```python
from build123d import *

# Parameters (mm, degrees)
CHAMFER1_SIZE  = 0.5
CHAMFER1_SIZE2 = 0.3
CHAMFER2_SIZE  = 0.5
CHAMFER2_SIZE2 = 0.75


with BuildPart() as part:
    # Sketch1 → Revolve1 (revolve)
    with BuildSketch(Plane.XY):
        Polygon((3.75, 0), (3.75, 1.16), (1.6, 1.16), (1.6, 3.45), (0.625, 3.45), (0.625, 6.44), (2.645, 6.44), (2.645, 14.44), (3.095, 14.44), (3.095, 5.95), (1.6, 5.95), (1.6, 4.45), (3.09, 4.45), (3.09, 1.77), (4.5, 1.77), (4.5, 0), align=None)
    revolve(axis=Axis((0, 0, 0), (0, 1, 0)))

    # Chamfer1
    chamfer1_edges = [part.edges().sort_by_distance(p)[0] for p in [
        (-2.645, 14.44, 0),
    ]]
    chamfer1_side = [part.faces().sort_by_distance(p)[0] for p in [
        (-2.645, 10.44, 0),
    ]]
    chamfer(chamfer1_edges, length=CHAMFER1_SIZE, length2=CHAMFER1_SIZE2, reference=chamfer1_side[0])

    # Chamfer2
    chamfer2_edges = [part.edges().sort_by_distance(p)[0] for p in [
        (-3.095, 5.95, 0),
    ]]
    chamfer2_side = [part.faces().sort_by_distance(p)[0] for p in [
        (-3.095, 10.195, 0),
    ]]
    chamfer(chamfer2_edges, length=CHAMFER2_SIZE, length2=CHAMFER2_SIZE2, reference=chamfer2_side[0])


solid = part.part
```
Can you work these out from the model? Positions are in its coordinate system, mm. A direction names the side the tool comes from. Give positions to 0.01 mm unless a question says otherwise; leave off trailing zeros. Write each loop counter-clockwise with the first axis right and the second up, starting at its lowest first coordinate (ties: lowest second). Pieces come first, ordered by that corner, then holes. Notation, with made-up numbers: (-35, 0.5) -> (12, 0.5) arc R17 ccw to (12, 12.5) -> close; hole circle Ø3 at (45.25, 80.5). An arc over 180 degrees is marked (long way). Write item = value, one per line.
(1) I'm going to push flat-ended pins straight in: P1, Ø3.5, axis at x = 0.5, z = -0.5, coming from the -Y side; P2, Ø1, axis at x = 2.5, z = -3.5, coming from the +Y side; P3, Ø2, axis at x = 0, z = 0, coming from the -Y side. Where does each tip first touch, or does it pass through?
Worked out:
P1 = 1.16
P2 = 1.77
P3 = 3.45
(2) Suppose I cut it at B-B on z = -3.25. Write out the boundary of the cut face in (x, y), then the cut area to 3 significant figures.
Worked out:
outline = (-3.11, 0) -> (-1.87, 0) -> (-1.87, 1.16) -> (1.87, 1.16) -> (1.87, 0) -> (3.11, 0) -> (3.11, 1.77) -> (-3.11, 1.77) -> close
area = 6.68 mm^2
(3) I need wall thicknesses on probe 1 along Z at (x, y) = (0, 4.8) (3 decimals); probe 2 along X at (y, z) = (0.8, 0). Which ranges of each line are inside material? Lowest first, please. Write a range as from..to.
Worked out:
probe_1 = -1.6..-0.625, 0.625..1.6
probe_2 = -4.5..-3.75, 3.75..4.5
(4) Suppose I cut it at C-C on x = 4. Write out the boundary of the cut face in (y, z).
Worked out:
outline = (0, -2.06) -> (1.77, -2.06) -> (1.77, 2.06) -> (0, 2.06) -> close
(5) Suppose I cut it at A-A on y = 9.75. Write out the boundary of the cut face in (x, z) (3 decimals), then the cut area to 3 significant figures.
Worked out:
outline = circle Ø6.19 at (0, 0); hole circle Ø5.29 at (0, 0)
area = 8.11 mm^2
(6) For faces 1 (the face through (-0.344, 10.242, -2.622)), 2 (the face through (-1.27, 2.32, 0.97)), 3 (the face through (0, 5.95, 2)), which set-ups out of +Z, -Z, +X, -X, +Y, -Y let a thin tool reach every point of the face, with its end or its side?
Worked out:
face_1 = +Y
face_2 = -Y
face_3 = none
(7) Thinking about a two-plate mould opening in Z: for faces 4 (the face through (-1.27, 5.19, 0.97)), 5 (the face through (3.1, 1.77, -1.1)), 6 (the face through (1, 3.45, 0)), which applies, released by +Z, released by -Z, zero draft, split by the parting line, or undercut?
Worked out:
face_4 = split by the parting line
face_5 = zero draft
face_6 = undercut
(8) Suppose I cut it at D-D on y = 2.25. Write out the boundary of the cut face in (x, z), then the cut area to 3 significant figures.
Worked out:
outline = circle Ø6.18 at (0, 0); hole circle Ø3.2 at (0, 0)
area = 22.0 mm^2
